Verification items for the finished model (mm, model axes). Give positions to 0.01 mm unless a question says otherwise; leave off trailing zeros. Write each loop counter-clockwise with the first axis right and the second up, starting at its lowest first coordinate (ties: lowest second). Pieces come first, ordered by that corner, then holes.
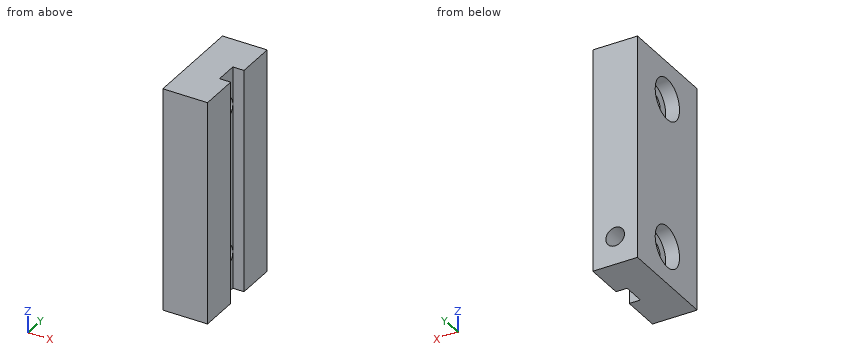
from build123d import *

# Parameters (mm, degrees)
SKETCH1_W                                = 60
SKETCH1_H                                = 10.5
BOSS_EXTRUDE1_DEPTH                      = 12
BOSS_EXTRUDE1_2_DEPTH                    = 12
SKETCH1_4_W                              = 60
SKETCH1_4_H                              = 6
BOSS_EXTRUDE2_DEPTH                      = 9
CBORE_FOR_M5_PAN_HEAD_SCREW1_D           = 6
CBORE_FOR_M5_PAN_HEAD_SCREW1_CBORE_D     = 11
CBORE_FOR_M5_PAN_HEAD_SCREW1_CBORE_DEPTH = 3.7
F_5_0_5_DIAMETER_HOLE17_D                = 5
F_5_0_5_DIAMETER_HOLE17_DEPTH            = 8.2
F_5_0_5_DIAMETER_HOLE17_TIP              = 1.502151548
F_5_0_5_DIAMETER_HOLE17_ON_FACE_2_D      = 5
F_5_0_5_DIAMETER_HOLE17_ON_FACE_2_DEPTH  = 8.2
F_5_0_5_DIAMETER_HOLE17_ON_FACE_2_TIP    = 1.502151548


with BuildPart() as part:
    # Sketch1 → Boss-Extrude1 (new body)
    with BuildSketch(Plane(origin=(0, 0, 0), x_dir=(0, 0, -1), z_dir=(1, 0, 0))):
        with Locations((0, 8.25)):
            Rectangle(SKETCH1_W, SKETCH1_H)
    extrude(amount=BOSS_EXTRUDE1_DEPTH)



with BuildPart() as body_2:
    # Sketch1 → Boss-Extrude1 2 (new body)
    with BuildSketch(Plane(origin=(0, 0, 0), x_dir=(0, 0, -1), z_dir=(1, 0, 0))):
        with Locations((0, -8.25)):
            Rectangle(SKETCH1_W, SKETCH1_H)
    extrude(amount=BOSS_EXTRUDE1_2_DEPTH)


with BuildPart() as part_1:
    add(part.part)

    add(body_2.part)  # Boss-Extrude2 merges body 2
    # Sketch1<4> → Boss-Extrude2 (add)
    with BuildSketch(Plane(origin=(0, 0, 0), x_dir=(0, 0, -1), z_dir=(1, 0, 0))):
        Rectangle(SKETCH1_4_W, SKETCH1_4_H)
    extrude(amount=BOSS_EXTRUDE2_DEPTH)

    # CBORE for M5 Pan Head Screw1 (through all)
    with Locations(Plane(origin=(0, 0, -20), x_dir=(0, 0, -1), z_dir=(-1, 0, 0))):
        with Locations((0, 0), (-40, 0)):
            CounterBoreHole(CBORE_FOR_M5_PAN_HEAD_SCREW1_D / 2, CBORE_FOR_M5_PAN_HEAD_SCREW1_CBORE_D / 2, CBORE_FOR_M5_PAN_HEAD_SCREW1_CBORE_DEPTH)

    # Ø5.0 (5) Diameter Hole17
    with Locations(Plane(origin=(6, 13.5, -22.5), x_dir=(0, 0, 1), z_dir=(0, 1, 0))):
        with Locations((0, 0)):
            Hole(F_5_0_5_DIAMETER_HOLE17_D / 2, depth=F_5_0_5_DIAMETER_HOLE17_DEPTH)
            with Locations((0, 0, -(F_5_0_5_DIAMETER_HOLE17_DEPTH + F_5_0_5_DIAMETER_HOLE17_TIP / 2))):  # 118° drill point
                Cone(0, F_5_0_5_DIAMETER_HOLE17_D / 2, F_5_0_5_DIAMETER_HOLE17_TIP, mode=Mode.SUBTRACT)

    # Ø5.0 (5) Diameter Hole17 on face 2
    with Locations(Plane(origin=(-4.960948742, 0, -17.906998739), x_dir=(0, 0, 1), z_dir=(0, 1, 0))):
        with Locations((0, 0), (0.436961169, -4.141332284)):
            Hole(F_5_0_5_DIAMETER_HOLE17_ON_FACE_2_D / 2, depth=F_5_0_5_DIAMETER_HOLE17_ON_FACE_2_DEPTH)
            with Locations((0, 0, -(F_5_0_5_DIAMETER_HOLE17_ON_FACE_2_DEPTH + F_5_0_5_DIAMETER_HOLE17_ON_FACE_2_TIP / 2))):  # 118° drill point
                Cone(0, F_5_0_5_DIAMETER_HOLE17_ON_FACE_2_D / 2, F_5_0_5_DIAMETER_HOLE17_ON_FACE_2_TIP, mode=Mode.SUBTRACT)


solid = part_1.part
Item 1: Sectioned sample at B-B on x = 10. Record the cut outline in (y, z), then the cut area to 3 significant figures.
Answer key:
outline: (-13.5, -30) - (-3, -30) - (-3, 30) - (-13.5, 30) - close; (3, -30) - (13.5, -30) - (13.5, 30) - (3, 30) - close
area: 1,260 mm2
Item 2: Depth check by flat-ended pin: pin 1 (5.5 mm diameter, centred on y = -0.5, z = -19, fed in from -X); pin 2 (5 mm diameter, centred on y = 2.5, z = -15.5, fed in from -X); pin 3 (3 mm diameter, centred on y = 1, z = -26.5, fed in from +X); pin 4 (5.5 mm diameter, centred on y = 0, z = -20, fed in from +X). Enter the tip coordinate at first touch or a pass-through.
Answer key:
pin 1: stops at x = 3.7
pin 2: stops at x = 0
pin 3: stops at x = 9
pin 4: passes through
Item 3: Sectioned sample at A-A on y = 0. Record the cut outline in (x, z).
Answer key:
outline: (0, -30) - (9, -30) - (9, -23) - (3.7, -23) - (3.7, -25.5) - (0, -25.5) - close; (0, -14.5) - (3.7, -14.5) - (3.7, -17) - (9, -17) - (9, 17) - (3.7, 17) - (3.7, 14.5) - (0, 14.5) - close; (0, 25.5) - (3.7, 25.5) - (3.7, 23) - (9, 23) - (9, 30) - (0, 30) - close
Item 4: Sectioned sample at D-D on z = 4. Record the cut outline in (x, y), then the cut area to 3 significant figures.
Answer key:
outline: (0, -13.5) - (12, -13.5) - (12, -3) - (9, -3) - (9, 3) - (12, 3) - (12, 13.5) - (0, 13.5) - close
area: 306 mm2
Item 5: Scan lines: line 1 along Y through (x, z) = (10.75, -17); line 2 along Y through (x, z) = (2.25, 20); line 3 along Z through (x, y) = (3.5, -1.25). Record each from-to range of solid material in increasing order.
Answer key:
line 1: y = -13.5 to -3, 3 to 13.5
line 2: y = -13.5 to -5.5, 5.5 to 13.5
line 3: z = -30 to -25.36, -14.64 to 14.64, 25.36 to 30
Item 6: Sectioned sample at C-C on y = 11. Record the cut outline in (x, z).
Answer key:
outline: (0, -30) - (12, -30) - (12, 30) - (0, 30) - close; hole circle Ø5 at (6, -22.5)
